```python
from build123d import *

# Parameters (mm, degrees)
BASE_FLANGE1_DEPTH         = 1
SKETCHED_START             = 31
SKETCHED_BEND1_DEPTH       = 178
SKETCHED_BEND1_2_DEPTH     = 793
SKETCHED_BEND1_3_OUTLINE_W = 793
SKETCHED_BEND1_3_OUTLINE_H = 1
SKETCHED_BEND1_3_DEPTH     = 29.234623369
SKETCHED_START_2           = 210.765376631
SKETCHED_BEND1_4_OUTLINE_W = 793
SKETCHED_BEND1_4_OUTLINE_H = 1
SKETCHED_BEND1_4_DEPTH     = 29.234623369
SKETCHED_BEND1_5_DEPTH     = 178
SKETCHED_BEND1_6_DEPTH     = 793
SKETCHED_BEND1_7_OUTLINE_W = 178
SKETCHED_BEND1_7_OUTLINE_H = 1
SKETCHED_BEND1_7_DEPTH     = 29.234623369
SKETCHED_START_3           = 825.765376631
SKETCHED_BEND1_8_OUTLINE_W = 178
SKETCHED_BEND1_8_OUTLINE_H = 1
SKETCHED_BEND1_8_DEPTH     = 29.234623369


# Read off the part's stored shape, not the designer's step: Sketched Bend1
# Sheet-metal steps are written as plain solids
with BuildPart() as part:
    # Sketch1 → Base-Flange1 (new body)
    with BuildSketch(Plane.XY):
        Polygon((0, 209), (31, 209), (31, 240), (824, 240), (824, 209), (855, 209), (855, 31), (824, 31), (824, 0), (31, 0), (31, 31), (0, 31), align=None)
    extrude(amount=-BASE_FLANGE1_DEPTH)

    # Sketched Bend1 outline → Sketched Bend1 (add)
    with BuildSketch(Plane(origin=(0, 0, 0), x_dir=(1, 0, 0), z_dir=(0, 1, 0)).offset(SKETCHED_START)):
        with BuildLine():
            Line((29.234623369, -0.7366), (29.234623369, -29.765376631))
            Line((29.234623369, -29.765376631), (30.234623369, -29.765376631))
            Line((30.234623369, -29.765376631), (30.234623369, -0.7366))
            ThreePointArc((30.234623369, -0.7366), (30.450368514, -0.215745145), (30.971223369, 0))
            Line((30.971223369, 0), (29.398582279, 0))
            ThreePointArc((29.398582279, 0), (29.276108612, -0.359286442), (29.234623369, -0.7366))
        make_face()
        with BuildLine():
            Line((825.601417721, 0), (824.028776631, 0))
            ThreePointArc((824.028776631, 0), (824.549631486, -0.215745145), (824.765376631, -0.7366))
            Line((824.765376631, -0.7366), (824.765376631, -29.765376631))
            Line((824.765376631, -29.765376631), (825.765376631, -29.765376631))
            Line((825.765376631, -29.765376631), (825.765376631, -0.7366))
            ThreePointArc((825.765376631, -0.7366), (825.723891388, -0.359286442), (825.601417721, 0))
        make_face()
    extrude(amount=SKETCHED_BEND1_DEPTH)

    # Sketched Bend1 2 outline → Sketched Bend1 2 (add)
    with BuildSketch(Plane.YZ.offset(SKETCHED_START)):
        with BuildLine():
            Line((209.028776631, 0), (210.601417721, 0))
            ThreePointArc((210.601417721, 0), (210.723891388, 0.359286442), (210.765376631, 0.7366))
            Line((210.765376631, 0.7366), (210.765376631, 29.765376631))
            Line((210.765376631, 29.765376631), (209.765376631, 29.765376631))
            Line((209.765376631, 29.765376631), (209.765376631, 0.7366))
            ThreePointArc((209.765376631, 0.7366), (209.549631486, 0.215745145), (209.028776631, 0))
        make_face()
        with BuildLine():
            ThreePointArc((29.234623369, 0.7366), (29.276108612, 0.359286442), (29.398582279, 0))
            Line((29.398582279, 0), (30.971223369, 0))
            ThreePointArc((30.971223369, 0), (30.450368514, 0.215745145), (30.234623369, 0.7366))
            Line((30.234623369, 0.7366), (30.234623369, 29.765376631))
            Line((30.234623369, 29.765376631), (29.234623369, 29.765376631))
            Line((29.234623369, 29.765376631), (29.234623369, 0.7366))
        make_face()
    extrude(amount=SKETCHED_BEND1_2_DEPTH)

    # Sketched Bend1 3 outline → Sketched Bend1 3 (cut)
    with BuildSketch(Plane(origin=(0, 0, 0), x_dir=(1, 0, 0), z_dir=(0, 1, 0))):
        with Locations((427.5, 0.5)):
            Rectangle(SKETCHED_BEND1_3_OUTLINE_W, SKETCHED_BEND1_3_OUTLINE_H)
    extrude(amount=SKETCHED_BEND1_3_DEPTH, mode=Mode.SUBTRACT)

    # Sketched Bend1 4 outline → Sketched Bend1 4 (cut)
    with BuildSketch(Plane(origin=(0, 0, 0), x_dir=(1, 0, 0), z_dir=(0, 1, 0)).offset(SKETCHED_START_2)):
        with Locations((427.5, 0.5)):
            Rectangle(SKETCHED_BEND1_4_OUTLINE_W, SKETCHED_BEND1_4_OUTLINE_H)
    extrude(amount=SKETCHED_BEND1_4_DEPTH, mode=Mode.SUBTRACT)

    # Sketched Bend1 5 outline → Sketched Bend1 5 (cut)
    with BuildSketch(Plane(origin=(0, 0, 0), x_dir=(1, 0, 0), z_dir=(0, 1, 0)).offset(SKETCHED_START)):
        with BuildLine():
            Line((0, 0), (29.398582279, 0))
            ThreePointArc((29.398582279, 0), (30.039397205, 0.728828115), (30.971223369, 1))
            Line((30.971223369, 1), (0, 1))
            Line((0, 1), (0, 0))
        make_face()
        with BuildLine():
            Line((855, 1), (824.028776631, 1))
            ThreePointArc((824.028776631, 1), (824.960602795, 0.728828115), (825.601417721, 0))
            Line((825.601417721, 0), (855, 0))
            Line((855, 0), (855, 1))
        make_face()
    extrude(amount=SKETCHED_BEND1_5_DEPTH, mode=Mode.SUBTRACT)

    # Sketched Bend1 6 outline → Sketched Bend1 6 (cut)
    with BuildSketch(Plane.YZ.offset(SKETCHED_START)):
        with BuildLine():
            ThreePointArc((210.601417721, 0), (209.960602795, -0.728828115), (209.028776631, -1))
            Line((209.028776631, -1), (240, -1))
            Line((240, -1), (240, 0))
            Line((240, 0), (210.601417721, 0))
        make_face()
        with BuildLine():
            Line((0, -1), (30.971223369, -1))
            ThreePointArc((30.971223369, -1), (30.039397205, -0.728828115), (29.398582279, 0))
            Line((29.398582279, 0), (0, 0))
            Line((0, 0), (0, -1))
        make_face()
    extrude(amount=SKETCHED_BEND1_6_DEPTH, mode=Mode.SUBTRACT)

    # Sketched Bend1 7 outline → Sketched Bend1 7 (cut)
    with BuildSketch(Plane.YZ):
        with Locations((120, -0.5)):
            Rectangle(SKETCHED_BEND1_7_OUTLINE_W, SKETCHED_BEND1_7_OUTLINE_H)
    extrude(amount=SKETCHED_BEND1_7_DEPTH, mode=Mode.SUBTRACT)

    # Sketched Bend1 8 outline → Sketched Bend1 8 (cut)
    with BuildSketch(Plane.YZ.offset(SKETCHED_START_3)):
        with Locations((120, -0.5)):
            Rectangle(SKETCHED_BEND1_8_OUTLINE_W, SKETCHED_BEND1_8_OUTLINE_H)
    extrude(amount=SKETCHED_BEND1_8_DEPTH, mode=Mode.SUBTRACT)


solid = part.part
```
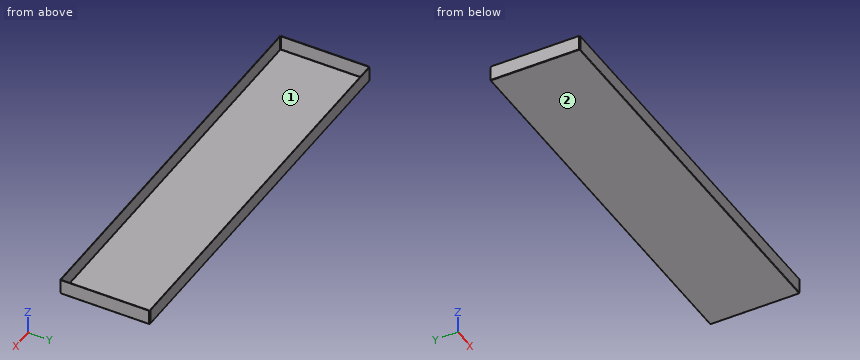
Input: part model. Units: mm. Frame: model coordinates. Face numbers are marked on the shaded views. Coordinates: 2 decimals unless noted, no trailing zeros. Loops run counter-clockwise (first coordinate to the right, second up) from the corner with the lowest first, then second, coordinate; pieces in that order, holes last.
Q1. Section A-A, the plane z = 17. Return the cut outline in (x, y), and give its area (3 significant figures).
Results are:
outline: (29.23, 31) - (30.23, 31) - (30.23, 209) - (29.23, 209) - close; (31, 29.23) - (824, 29.23) - (824, 30.23) - (31, 30.23) - close; (31, 209.77) - (824, 209.77) - (824, 210.77) - (31, 210.77) - close; (824.77, 31) - (825.77, 31) - (825.77, 209) - (824.77, 209) - close
area: 1,940 mm2
Q2. Contact query for flat-ended pins moving along their axis: pin 1 (0.5 mm diameter, centred on x = 825, z = 10.5, fed in from -Y); pin 2 (1 mm diameter, centred on x = 673, y = 95.5, fed in from +Z); pin 3 (1.4 mm diameter, centred on y = 30, z = 20.5, fed in from -X). Output: stop coordinate, or through.
Results are:
pin 1: stops at y = 31
pin 2: stops at z = 0
pin 3: stops at x = 31
Q3. Section B-B, the plane x = 238. Return the cut outline in (y, z), and give its area (3 significant figures).
Results are:
outline: (29.23, 0.74) arc R1.74 ccw to (30.97, -1) - (209.03, -1) arc R1.74 ccw to (210.77, 0.74) - (210.77, 29.77) - (209.77, 29.77) - (209.77, 0.74) arc R0.74 cw to (209.03, 0) - (30.97, 0) arc R0.74 cw to (30.23, 0.74) - (30.23, 29.77) - (29.23, 29.77) - close
area: 240 mm2
Q4. Section C-C, the plane y = 147. Return the cut outline in (x, z).
Results are:
outline: (29.23, 0.74) arc R1.74 ccw to (30.97, -1) - (824.03, -1) arc R1.74 ccw to (825.77, 0.74) - (825.77, 29.77) - (824.77, 29.77) - (824.77, 0.74) arc R0.74 cw to (824.03, 0) - (30.97, 0) arc R0.74 cw to (30.23, 0.74) - (30.23, 29.77) - (29.23, 29.77) - close
Q5. Line query: line 1 along X through (y, z) = (171, 20); line 2 along Y through (x, z) = (221.5, 25); line 3 along Z through (x, y) = (171, 97.5). Output: solid intervals per line, ascending.
Results are:
line 1: x = 29.23 to 30.23, 824.77 to 825.77
line 2: y = 29.23 to 30.23, 209.77 to 210.77
line 3: z = -1 to 0
Q6. Mould query, pull axis Y, two halves, no side actions, for the marked faces 1 and 2. Classes: +Y half, -Y half, draft (parallel to the pull), parting line (faces both ways), or undercut.
Results are:
face 1: undercut
face 2: draft
